```python
from build123d import *

# Parameters (mm, degrees)
BASESTEELANGLE_DEPTH = 50.8


with BuildPart() as part:
    # Sketch1 → BaseSteelAngle (new body, symmetric)
    with BuildSketch(Plane.XY):
        with BuildLine():
            Line((0, 0), (0, 19.05))
            Line((0, 19.05), (0.00508, 19.05))
            ThreePointArc((0.00508, 19.05), (2.246551928, 18.121551928), (3.175, 15.88008))
            Line((3.175, 15.88008), (3.175, 7.9375))
            ThreePointArc((3.175, 7.9375), (4.569903955, 4.569903955), (7.9375, 3.175))
            Line((7.9375, 3.175), (15.88008, 3.175))
            ThreePointArc((15.88008, 3.175), (18.121551928, 2.246551928), (19.05, 0.00508))
            Line((19.05, 0.00508), (19.05, 0))
            Line((19.05, 0), (0, 0))
        make_face()
    extrude(amount=BASESTEELANGLE_DEPTH, both=True)

    # Sketch4 → 5/16 (0.3125) Diameter Hole2 (revolve, cut)
    with BuildSketch(Plane(origin=(9.525, 3.175, 39.8), x_dir=(0, 0, 1), z_dir=(1, 0, 0))):
        Polygon((0, 0), (0, 21.434665582), (3.96875, 19.05), (3.96875, 0), align=None)
    f_5_16_0_3125_diameter_hole2 = revolve(axis=Axis((9.525, 9.525, 39.8), (0, -1, 0)), mode=Mode.SUBTRACT)

    # Mirror1: 5/16 (0.3125) Diameter Hole2 across plane
    add(f_5_16_0_3125_diameter_hole2.mirror(Plane.XY), mode=Mode.SUBTRACT)

    # Sketch6 → 5/16 (0.3125) Diameter Hole3 (revolve, cut)
    with BuildSketch(Plane(origin=(3.175, 9.525, 39.8), x_dir=(0, 0, -1), z_dir=(0, 1, 0))):
        Polygon((0, 0), (0, 21.434665582), (3.96875, 19.05), (3.96875, 0), align=None)
    f_5_16_0_3125_diameter_hole3 = revolve(axis=Axis((9.525, 9.525, 39.8), (-1, 0, 0)), mode=Mode.SUBTRACT)

    # Mirror2: 5/16 (0.3125) Diameter Hole3 across plane
    add(f_5_16_0_3125_diameter_hole3.mirror(Plane.XY), mode=Mode.SUBTRACT)


solid = part.part
```
Read the model definition and answer for the solid it produces. Units are mm, in the model's axes. A direction names the side the tool comes from. Coordinates: 2 decimals unless noted, no trailing zeros. Write each loop counter-clockwise with the first axis right and the second up, starting at its lowest first coordinate (ties: lowest second). Pieces come first, ordered by that corner, then holes. Notation, with made-up numbers: (-34.5, 82.5) -> (-13.5, 82.5) arc R9 ccw to (-13.5, 91.5) -> close; hole circle Ø2 at (38.5, 4). An arc over 180 degrees is marked (long way). Write item = value, one per line.
(1) Which of the six approach directions +Z, -Z, +X, -X, +Y, -Y give full straight-line access (tool end or side, diameter ignored) to faces 5 (the face through (1.61, 11.94, -42.95)), 6 (the face through (6.7, 3.175, -39.7)), 7 (the face through (10, 0, 1))?
From the geometry:
face_5 = -X
face_6 = -Y
face_7 = +Z, -Z, +X, -X, -Y
(2) Section A-A on z = -39.8 is taken. Count the separate pieces of the cut face and the enclosed holes in it, plus the area to 3 significant figures.
From the geometry:
separate_pieces = 3
enclosed_holes = 0
area = 61.0 mm2
(3) Section C-C on y = 1.5 is taken. Write down the section's boundary in (x, z) (1 decimal).
From the geometry:
outline = (0, -50.8) -> (18.7, -50.8) -> (18.7, 50.8) -> (0, 50.8) -> close; hole circle Ø7.9 at (9.5, -39.8); hole circle Ø7.9 at (9.5, 39.8)
(4) Section D-D on y = 15 is taken. Write down the section's boundary in (x, z) (3 decimals), plus the area to 3 significant figures.
From the geometry:
outline = (0, -50.8) -> (3.175, -50.8) -> (3.175, 50.8) -> (0, 50.8) -> close
area = 323 mm2
(5) Given pin 1 Ø5 at (x, z) = (9.525, 39.8) entering from +Y; pin 2 Ø2.5 at (y, z) = (13.5, -14) entering from +X (3 decimals); pin 3 Ø7 at (y, z) = (9.525, -39.8) entering from +X, each flat-ended and moving along its own axis, determine where each tip first touches the part or whether it passes through.
From the geometry:
pin_1 = 3.26
pin_2 = 3.175
pin_3 = 3.58
(6) Straight lines are drawn through the part: L1, parallel to Y at x = 15.5, z = -27.5 (3 decimals); L2, parallel to Z at x = 2.5, y = 10.5. For each, find the intervals that lie inside material, in ascending order. Write a range as from..to.
From the geometry:
L1 = 0..3.175
L2 = -50.8..-43.65, -35.95..35.95, 43.65..50.8
(7) For a pull along X with two mould halves and no side action, classify faces 1 (the face through (3.175, 12, 1)), 2 (the face through (12, 3.175, 1)), 3 (the face through (11.94, 1.61, 36.65)), 4 (the face through (11.94, 1.61, -36.65)) as +X half, -X half, draft (parallel to the pull), parting line (faces both ways), or undercut.
From the geometry:
face_1 = +X half
face_2 = draft
face_3 = undercut
face_4 = undercut
